from build123d import *

# Parameters (mm, degrees)
CUT_EXTRUDE1_DEPTH      = 212.88306668
BOSS_EXTRUDE2_DEPTH     = 139.7
SKETCH9_R               = 35.95202499
BOSS_EXTRUDE3_DEPTH     = 4
CUT_EXTRUDE2_DEPTH      = 4
SKETCH11_W              = 10
SKETCH11_H              = 34
CUT_EXTRUDE3_DEPTH      = 15
RASPBERRY_PI_5_DEPTH    = 4
GPS_SLOT_DEPTH          = 5.1
SKETCH14_W              = 10
SKETCH14_H              = 16
MPU_DEPTH               = 434.220724454
ALTIMETER_DEPTH         = 434.220724454
ALTIMETER_DEPTH_BACK    = 3.54
SKETCH15_W              = 20
SKETCH15_H              = 15.34
SKETCH16_W              = 62.2
SKETCH16_H              = 25.5
PCA9685_DEPTH           = 2
SKETCH17_W              = 50
SKETCH17_H              = 27
ESP_32_1_DEPTH          = 5
SKETCH18_W              = 55
SKETCH18_H              = 30.1
BATTERY_1_DEPTH         = 3.5
SKETCH21_W              = 55
SKETCH21_H              = 30.1
BATTERY_2_DEPTH         = 3.5
SKETCH24_W              = 50
SKETCH24_H              = 27
ESP_32_MESHTASTIC_DEPTH = 5
SKETCH25_W              = 21.1
SKETCH25_H              = 43.1
STEP_DOWN_DEPTH         = 1
SKETCH26_W              = 50
SKETCH26_H              = 27
ESP_32_2_DEPTH          = 5
BOSS_EXTRUDE4_START     = -120
SKETCH27_R              = 36.3
SKETCH27_R_2            = 30
BOSS_EXTRUDE4_DEPTH     = 7
CUT_EXTRUDE4_START      = -127
SKETCH29_R              = 36.3
CUT_EXTRUDE4_DEPTH      = 226.865446219
SKETCH30_W              = 4
SKETCH30_H              = 24.4
CUT_EXTRUDE5_DEPTH      = 5.1
CUT_EXTRUDE6_REACH      = 140.027
SKETCH31_R              = 2.55


with BuildPart() as part:
    # Sketch3 → Revolve1 (revolve)
    with BuildSketch(Plane.XY):
        with BuildLine():
            Line((285.74876522, 39.710021262), (285.74876522, 3.757996272))
            Line((285.74876522, 3.757996272), (80.74876522, 3.757996272))
            Line((80.74876522, 3.757996272), (80.74876522, 19.634316044))
            add(Edge.make_bspline(
                [(80.74876522, 19.634316044), (82.347112552, 19.950400666), (85.636412123, 20.593859316), (92.311794173, 21.870421625), (109.164486257, 24.943674568), (127.867996046, 27.977765645), (146.633052135, 30.604670801), (163.733801994, 32.658467989), (174.004488004, 33.801497199), (184.284802392, 34.855212792), (194.57611333, 35.797171826), (204.876878825, 36.627240946), (213.466527777, 37.244314669), (220.34120026, 37.693162367), (227.218898943, 38.097179671), (233.238636081, 38.411453209), (238.400481516, 38.652791264), (242.701722554, 38.8352093), (246.145182192, 38.969923968), (249.584994627, 39.093417446), (253.03241088, 39.20568842), (256.467961578, 39.306735697), (259.924132141, 39.396558203), (263.346991762, 39.475154984), (266.82565511, 39.542525204), (270.211898057, 39.598668148), (273.756466178, 39.643583219), (276.60509147, 39.673059099), (279.43950326, 39.691306197), (281.597603414, 39.703938851), (283.942998009, 39.708617629), (285.03032454, 39.710021262), (285.74876522, 39.710021262)],
                knots=[0.322773044, 0.322773044, 0.322773044, 0.322773044, 0.322773044, 0.341563488, 0.3614269, 0.401153715, 0.520334158, 0.56006097, 0.579924379, 0.599787787, 0.639514601, 0.679241414, 0.699104823, 0.718968231, 0.738831638, 0.758695045, 0.778558452, 0.788490156, 0.798421859, 0.808353563, 0.818285267, 0.828216971, 0.838148675, 0.848080378, 0.858012082, 0.867943786, 0.87787549, 0.887807193, 0.897738897, 0.902704749, 0.9076706, 0.917602304, 0.917602304, 0.917602304, 0.917602304, 0.917602304], degree=4))
        make_face()
    revolve(axis=Axis((285.74876522, 3.757996272, 0), (-1, 0, 0)))

    # Sketch6 → Cut-Extrude1 (cut, through all)
    with BuildSketch(Plane(origin=(285.74876522, 0, 0), x_dir=(0, 0, -1), z_dir=(1, 0, 0))):
        with BuildLine():
            Line((-5, -31.844645496), (-5, 39.36063804))
            ThreePointArc((-5, 39.360638041), (-35.95202499, 3.757996272), (-5, -31.844645496))
        make_face()
        with BuildLine():
            ThreePointArc((35.95202499, 3.757996272), (27.132160123, 27.346001444), (5, 39.36063804))
            Line((5, 39.36063804), (5, -31.844645496))
            ThreePointArc((5, -31.844645496), (27.132160123, -19.830008899), (35.95202499, 3.757996272))
        make_face()
    extrude(amount=-CUT_EXTRUDE1_DEPTH, mode=Mode.SUBTRACT)

    # Sketch8 → Boss-Extrude2 (add)
    with BuildSketch(Plane(origin=(285.74876522, 0, 0), x_dir=(0, 0, -1), z_dir=(1, 0, 0))):
        with BuildLine():
            Line((5, -31.844645496), (5, 39.360638041))
            ThreePointArc((5, 39.360638041), (0, 39.710021262), (-5, 39.360638041))
            Line((-5, 39.360638041), (-5, -31.844645496))
            ThreePointArc((-5, -31.844645496), (0, -32.194028718), (5, -31.844645496))
        make_face()
    extrude(amount=BOSS_EXTRUDE2_DEPTH)

    # Sketch9 → Boss-Extrude3 (add)
    with BuildSketch(Plane(origin=(425.44876522, 0, 0), x_dir=(0, 0, -1), z_dir=(1, 0, 0))):
        with Locations(Location((0, 3.757996272, 0), (0, 0, 262.00572083))):
            Circle(SKETCH9_R)
    extrude(amount=BOSS_EXTRUDE3_DEPTH)

    # Sketch10 → Cut-Extrude2 (cut)
    with BuildSketch(Plane(origin=(429.44876522, 0, 0), x_dir=(0, 0, -1), z_dir=(1, 0, 0))):
        Polygon((-17, -4.442003728), (-17, 11.957996272), (-8.2, 20.757996272), (8.2, 20.757996272), (17, 11.957996272), (17, -4.442003728), (8.2, -13.242003728), (-8.2, -13.242003728), align=None)
    extrude(amount=-CUT_EXTRUDE2_DEPTH, mode=Mode.SUBTRACT)

    # Sketch11 → Cut-Extrude3 (cut)
    with BuildSketch(Plane(origin=(425.44876522, 0, 0), x_dir=(0, 0, -1), z_dir=(1, 0, 0))):
        with Locations((0, 3.757996272)):
            Rectangle(SKETCH11_W, SKETCH11_H)
    extrude(amount=-CUT_EXTRUDE3_DEPTH, mode=Mode.SUBTRACT)

    # Sketch12 → Raspberry Pi 5 (cut)
    with BuildSketch(Plane.XY.offset(5)):
        with BuildLine():
            Line((407.44876522, -24.255570554), (321.24876522, -24.255570554))
            ThreePointArc((321.24876522, -24.255570554), (320.541658439, -23.962677335), (320.24876522, -23.255570554))
            Line((320.24876522, -23.255570554), (320.24876522, 30.944429446))
            ThreePointArc((320.24876522, 30.944429446), (320.541658439, 31.651536227), (321.24876522, 31.944429446))
            Line((321.24876522, 31.944429446), (407.44876522, 31.944429446))
            ThreePointArc((407.44876522, 31.944429446), (408.155872001, 31.651536227), (408.44876522, 30.944429446))
            Line((408.44876522, 30.944429446), (408.44876522, -23.255570554))
            ThreePointArc((408.44876522, -23.255570554), (408.155872001, -23.962677335), (407.44876522, -24.255570554))
        make_face()
    extrude(amount=-RASPBERRY_PI_5_DEPTH, mode=Mode.SUBTRACT)

    # Sketch13 → GPS Slot (cut)
    with BuildSketch(Plane.XY.offset(5)):
        with BuildLine():
            Line((294.985699539, 8.990821657), (262.335699539, 8.990821657))
            ThreePointArc((262.335699539, 8.990821657), (261.628592757, 9.283714876), (261.335699539, 9.990821657))
            Line((261.335699539, 9.990821657), (261.335699539, 33.590821657))
            ThreePointArc((261.335699539, 33.590821657), (261.628592757, 34.297928438), (262.335699539, 34.590821657))
            Line((262.335699539, 34.590821657), (294.985699539, 34.590821657))
            ThreePointArc((294.985699539, 34.590821657), (295.69280632, 34.297928438), (295.985699539, 33.590821657))
            Line((295.985699539, 33.590821657), (295.985699539, 9.990821657))
            ThreePointArc((295.985699539, 9.990821657), (295.69280632, 9.283714876), (294.985699539, 8.990821657))
        make_face()
    extrude(amount=-GPS_SLOT_DEPTH, mode=Mode.SUBTRACT)

    # Sketch14 → MPU (cut, through all)
    with BuildSketch(Plane.XY.offset(5)):
        with Locations((277.879699021, -20.106936119)):
            Rectangle(SKETCH14_W, SKETCH14_H)
    extrude(amount=-MPU_DEPTH, mode=Mode.SUBTRACT)

    # Sketch15 → Altimeter (cut, two sides: drawn at the far end of the back side and taken through both)
    with BuildSketch(Plane.XY.offset(5).offset(-ALTIMETER_DEPTH_BACK)):
        with Locations((285.717294066, -1.841089471)):
            Rectangle(SKETCH15_W, SKETCH15_H)
    extrude(amount=ALTIMETER_DEPTH + ALTIMETER_DEPTH_BACK, mode=Mode.SUBTRACT)

    # Sketch16 → PCA9685 (cut)
    with BuildSketch(Plane.XY.offset(5)):
        with Locations((132.808150825, 3.59036767)):
            Rectangle(SKETCH16_W, SKETCH16_H)
    extrude(amount=-PCA9685_DEPTH, mode=Mode.SUBTRACT)

    # Sketch17 → ESP-32 (1) (cut)
    with BuildSketch(Plane.XY.offset(5)):
        with Locations((233.402571461, -10.513286129)):
            Rectangle(SKETCH17_W, SKETCH17_H)
    extrude(amount=-ESP_32_1_DEPTH, mode=Mode.SUBTRACT)

    # Sketch18 → Battery 1 (cut)
    with BuildSketch(Plane(origin=(0, 0, -5), x_dir=(-1, 0, 0), z_dir=(0, 0, -1))):
        with Locations((-377.94876522, 19.967269146)):
            Rectangle(SKETCH18_W, SKETCH18_H)
    extrude(amount=-BATTERY_1_DEPTH, mode=Mode.SUBTRACT)

    # Sketch21 → Battery 2 (cut)
    with BuildSketch(Plane(origin=(0, 0, -5), x_dir=(-1, 0, 0), z_dir=(0, 0, -1))):
        with Locations((-377.94876522, -12.451276601)):
            Rectangle(SKETCH21_W, SKETCH21_H)
    extrude(amount=-BATTERY_2_DEPTH, mode=Mode.SUBTRACT)

    # Sketch24 → ESP-32 (Meshtastic) (cut)
    with BuildSketch(Plane(origin=(0, 0, -5), x_dir=(-1, 0, 0), z_dir=(0, 0, -1))):
        with Locations((-233.841762832, 18.555689361)):
            Rectangle(SKETCH24_W, SKETCH24_H)
    extrude(amount=-ESP_32_MESHTASTIC_DEPTH, mode=Mode.SUBTRACT)

    # Sketch25 → Step Down (cut)
    with BuildSketch(Plane(origin=(0, 0, -5), x_dir=(-1, 0, 0), z_dir=(0, 0, -1))):
        with Locations((-323.977591294, 5.876880331)):
            Rectangle(SKETCH25_W, SKETCH25_H)
    extrude(amount=-STEP_DOWN_DEPTH, mode=Mode.SUBTRACT)

    # Sketch26 → ESP-32 (2) (cut)
    with BuildSketch(Plane(origin=(0, 0, -5), x_dir=(-1, 0, 0), z_dir=(0, 0, -1))):
        with Locations((-165.478674332, 3.198326217)):
            Rectangle(SKETCH26_W, SKETCH26_H)
    extrude(amount=-ESP_32_2_DEPTH, mode=Mode.SUBTRACT)

    # Sketch27 → Boss-Extrude4 (add)
    with BuildSketch(Plane(origin=(429.44876522, 0, 0), x_dir=(0, 0, -1), z_dir=(1, 0, 0)).offset(BOSS_EXTRUDE4_START)):
        with Locations((0, 3.757996272)):
            Circle(SKETCH27_R)
        with Locations((0, 3.757996272)):
            Circle(SKETCH27_R_2, mode=Mode.SUBTRACT)
    extrude(amount=-BOSS_EXTRUDE4_DEPTH)

    # Sketch29 → Cut-Extrude4 (cut, through all)
    with BuildSketch(Plane(origin=(429.44876522, 0, 0), x_dir=(0, 0, -1), z_dir=(1, 0, 0)).offset(CUT_EXTRUDE4_START)):
        with Locations((0, 3.757996272)):
            Circle(SKETCH29_R)
    extrude(amount=-CUT_EXTRUDE4_DEPTH, mode=Mode.SUBTRACT)

    # Sketch30 → Cut-Extrude5 (cut)
    with BuildSketch(Plane.ZY.offset(-302.44876522)):
        with Locations((0, 3.757996272)):
            Rectangle(SKETCH30_W, SKETCH30_H)
    extrude(amount=-CUT_EXTRUDE5_DEPTH, mode=Mode.SUBTRACT)

    # Sketch31 → Cut-Extrude6 (cut, up to next)
    with BuildSketch(Plane(origin=(429.44876522, 0, 0), x_dir=(0, 0, -1), z_dir=(1, 0, 0)), mode=Mode.PRIVATE) as cut_extrude6_sk1:
        with Locations((20.859650045, 24.617646317)):
            Circle(SKETCH31_R)
    cut_extrude6_tool1 = extrude(cut_extrude6_sk1.sketch, amount=-CUT_EXTRUDE6_REACH, mode=Mode.PRIVATE) & part.part
    # Sketch31 → Cut-Extrude6 (cut, up to next)
    with BuildSketch(Plane(origin=(429.44876522, 0, 0), x_dir=(0, 0, -1), z_dir=(1, 0, 0)), mode=Mode.PRIVATE) as cut_extrude6_sk2:
        with Locations((-20.859650045, 24.617646317)):
            Circle(SKETCH31_R)
    cut_extrude6_tool2 = extrude(cut_extrude6_sk2.sketch, amount=-CUT_EXTRUDE6_REACH, mode=Mode.PRIVATE) & part.part
    # Sketch31 → Cut-Extrude6 (cut, up to next)
    with BuildSketch(Plane(origin=(429.44876522, 0, 0), x_dir=(0, 0, -1), z_dir=(1, 0, 0)), mode=Mode.PRIVATE) as cut_extrude6_sk3:
        with Locations((-20.859650045, -17.101653773)):
            Circle(SKETCH31_R)
    cut_extrude6_tool3 = extrude(cut_extrude6_sk3.sketch, amount=-CUT_EXTRUDE6_REACH, mode=Mode.PRIVATE) & part.part
    # Sketch31 → Cut-Extrude6 (cut, up to next)
    with BuildSketch(Plane(origin=(429.44876522, 0, 0), x_dir=(0, 0, -1), z_dir=(1, 0, 0)), mode=Mode.PRIVATE) as cut_extrude6_sk4:
        with Locations((20.859650045, -17.101653773)):
            Circle(SKETCH31_R)
    cut_extrude6_tool4 = extrude(cut_extrude6_sk4.sketch, amount=-CUT_EXTRUDE6_REACH, mode=Mode.PRIVATE) & part.part
    add(cut_extrude6_tool1.solids().sort_by_distance((429.448765, 24.617646, -20.85965))[0], mode=Mode.SUBTRACT)
    add(cut_extrude6_tool2.solids().sort_by_distance((429.448765, 24.617646, 20.85965))[0], mode=Mode.SUBTRACT)
    add(cut_extrude6_tool3.solids().sort_by_distance((429.448765, -17.101654, 20.85965))[0], mode=Mode.SUBTRACT)
    add(cut_extrude6_tool4.solids().sort_by_distance((429.448765, -17.101654, -20.85965))[0], mode=Mode.SUBTRACT)


solid = part.part
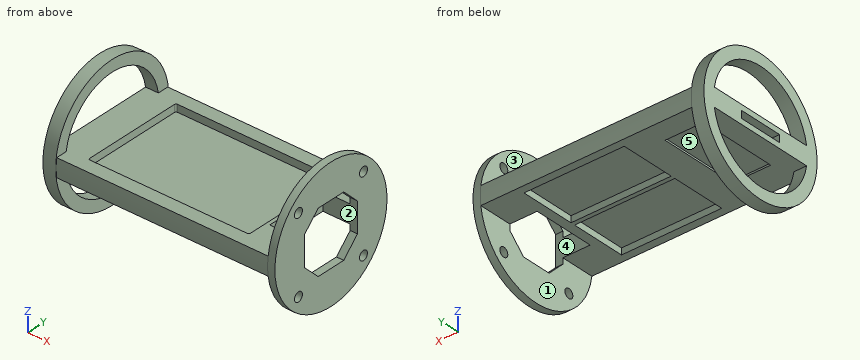
For this review, take the finished solid that the model builds, in its own axes (mm). Face numbers are marked on the shaded views. A direction names the side the tool comes from. Give positions to 0.01 mm unless a question says otherwise; leave off trailing zeros. Loops run counter-clockwise (first coordinate to the right, second up) from the corner with the lowest first, then second, coordinate; pieces in that order, holes last. Notation, with made-up numbers: (84.25, 68) -> (113.25, 68) arc R12 ccw to (113.25, 89) -> close; hole circle Ø5 at (35, 60). An arc over 180 degrees is marked (long way). One line per question, with ' | ' between items.
1) The part is to be moulded in two halves that separate along Y. For the marked faces 1 and 2, say which applies: +Y half, -Y half, draft (parallel to the pull), parting line (faces both ways), or undercut.
Resolved:
face 1: draft | face 2: undercut
2) We need section A-A (x = 402). Write out the cut boundary in (y, z).
Resolved:
outline: (-31.84, -5) -> (-27.5, -5) -> (-27.5, -1.5) -> (2.6, -1.5) -> (2.6, -5) -> (4.92, -5) -> (4.92, -1.5) -> (35.02, -1.5) -> (35.02, -5) -> (39.36, -5) arc R35.95 ccw to (39.36, 5) -> (31.94, 5) -> (31.94, 1) -> (-24.26, 1) -> (-24.26, 5) -> (-31.84, 5) arc R35.95 ccw to start
3) We need section C-C (z = 28). Write out the cut boundary in (x, y), plus the area to 3 significant figures.
Resolved:
outline: (302.45, -19.34) -> (309.45, -19.34) -> (309.45, -7.01) -> (302.45, -7.01) -> close; (302.45, 14.53) -> (309.45, 14.53) -> (309.45, 26.86) -> (302.45, 26.86) -> close; (425.45, -18.79) -> (429.45, -18.79) -> (429.45, 26.31) -> (425.45, 26.31) -> close | area: 353 mm2
4) To check wall thickness, follow probe 1 along X at (y, z) = (13.5, -29.5); probe 2 along Y at (x, z) = (380.5, -2); probe 3 along Z at (x, y) = (410, 5). State the ranges of each line that lie inside material, in increasing order.
Resolved:
probe 1: x = 302.45 to 309.45, 425.45 to 429.45 | probe 2: y = -32.14 to -27.5, 2.6 to 4.92, 35.02 to 39.65 | probe 3: z = -5 to 5
5) We need section B-B (z = -26.5). Write out the cut boundary in (x, y), plus the area to 3 significant figures.
Resolved:
outline: (302.45, -21.05) -> (309.45, -21.05) -> (309.45, -10.3) -> (302.45, -10.3) -> close; (302.45, 17.82) -> (309.45, 17.82) -> (309.45, 28.57) -> (302.45, 28.57) -> close; (425.45, -20.54) -> (429.45, -20.54) -> (429.45, 28.05) -> (425.45, 28.05) -> close | area: 345 mm2
6) For the marked faces 3, 4 and 5, list the 3-axis set-ups (+Z, -Z, +X, -X, +Y, -Y) from which the entire face can be reached by the end or side of a thin tool; tool diameter is ignored.
Resolved:
face 3: +Z, +Y, -Y | face 4: +X | face 5: -Z
7) We need section D-D (y = -6). Give the number of separate pieces and of enclosed holes in the cut face, plus the area to 3 significant figures.
Resolved:
separate pieces: 5 | enclosed holes: 0 | area: 739 mm2
8) Insertion check: pin 1 Ø1.8 at (x, z) = (367, -4) entering from +Y; pin 2 Ø1.2 at (x, y) = (427.5, 7) entering from +Z; pin 3 Ø2.5 at (x, y) = (305, 3) entering from -Z; pin 4 Ø2 at (y, z) = (9, 0) entering from -X. Each pin has a flat end and moves straight along its axis. Give the tip position at first contact, or say it passes through.
Resolved:
pin 1: stops at y = 39.58 | pin 2: stops at z = 35.85 | pin 3: stops at z = -36.3 | pin 4: stops at x = 307.55
